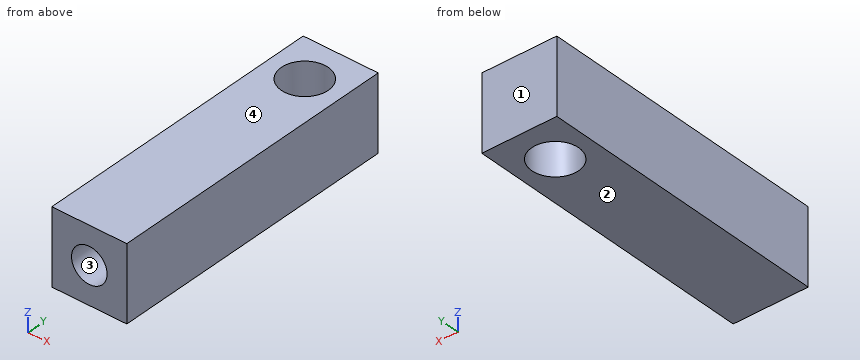
```python
from build123d import *

# Parameters (mm, degrees)
SKETCH_W        = 16
SKETCH_H        = 16
PAD_DEPTH       = 63
SKETCH001_R     = 5
POCKET_DEPTH    = 16
SKETCH002_R     = 3.8
POCKET001_DEPTH = 10


with BuildPart() as part:
    # Sketch → Pad (new body)
    with BuildSketch(Plane.XZ):
        Rectangle(SKETCH_W, SKETCH_H)
    extrude(amount=PAD_DEPTH)

    # Sketch001 → Pocket (cut)
    with BuildSketch(Plane(origin=(0, 0, 8), x_dir=(-1, 0, 0), z_dir=(0, 0, 1))):
        with Locations((0, 9)):
            Circle(SKETCH001_R)
    extrude(amount=-POCKET_DEPTH, mode=Mode.SUBTRACT)

    # Sketch002 → Pocket001 (cut)
    with BuildSketch(Plane.XZ.offset(63)):
        Circle(SKETCH002_R)
    extrude(amount=-POCKET001_DEPTH, mode=Mode.SUBTRACT)


solid = part.part
```
Geometry: final body of the model. Coordinates: model frame, mm. Face numbers are marked on the shaded views. Round coordinates to 2 decimals unless told otherwise and drop trailing zeros. Order: outer loops, then holes, each group sorted by start corner. A loop starts at its lowest first (then second) coordinate and runs counter-clockwise, first axis right, second up. Notation, with made-up numbers: (38, -22) -> (90, -22) arc R32 ccw to (90, 16) -> close; hole circle Ø8 at (61, 55). An arc over 180 degrees is marked (long way). Use CSV: the item, a comma, the result in double quotes. Start each with the question number.
1) Section D-D (z = 6.25). Return the cut outline in (x, y), and give its area (3 significant figures).
2) Section A-A (x = 0). Return the cut outline in (y, z).
3) Material intervals for line 1 along Y through (x, z) = (0, 2); line 2 along Z through (x, y) = (0, -58.75); line 3 along Y through (x, z) = (0, 4), sorted ascending. Write a range as from..to.
4) Section C-C (z = 0). Return the cut outline in (x, y).
5) Section B-B (y = -9). Return the cut outline in (x, z).
6) Draft query along Z for the marked faces 1, 2, 3 and 4. Return one class per face: +Z half, -Z half, draft (parallel to the pull), parting line (faces both ways), or undercut.
Returned:
1,outline,"(-8, -63) -> (8, -63) -> (8, 0) -> (-8, 0) -> close; hole circle Ø10 at (0, -9)"
1,area,"929 mm²"
2,outline,"(-63, -8) -> (-14, -8) -> (-14, 8) -> (-63, 8) -> (-63, 3.8) -> (-53, 3.8) -> (-53, -3.8) -> (-63, -3.8) -> close; (-4, -8) -> (0, -8) -> (0, 8) -> (-4, 8) -> close"
3,line 1,"y = -53..-14, -4..0"
3,line 2,"z = -8..-3.8, 3.8..8"
3,line 3,"y = -63..-14, -4..0"
4,outline,"(-8, -63) -> (-3.8, -63) -> (-3.8, -53) -> (3.8, -53) -> (3.8, -63) -> (8, -63) -> (8, 0) -> (-8, 0) -> close; hole circle Ø10 at (0, -9)"
5,outline,"(-8, -8) -> (-5, -8) -> (-5, 8) -> (-8, 8) -> close; (5, -8) -> (8, -8) -> (8, 8) -> (5, 8) -> close"
6,face 1,"draft"
6,face 2,"-Z half"
6,face 3,"undercut"
6,face 4,"+Z half"
